Study the drawing (mm; zero at the part's minimum x, y, z) and answer. A direction names the side the tool comes from. Give positions to 0.01 mm unless a question says otherwise; leave off trailing zeros. Write each loop counter-clockwise with the first axis right and the second up, starting at its lowest first coordinate (ties: lowest second). Pieces come first, ordered by that corner, then holes. Notation, with made-up numbers: (19, 30.5) - (46, 30.5) arc R34 cw to (46, 65.5) - close; hole circle Ø7 at (76, -25.75). An arc over 180 degrees is marked (long way). Return JSON: item names as keys, results as strings.
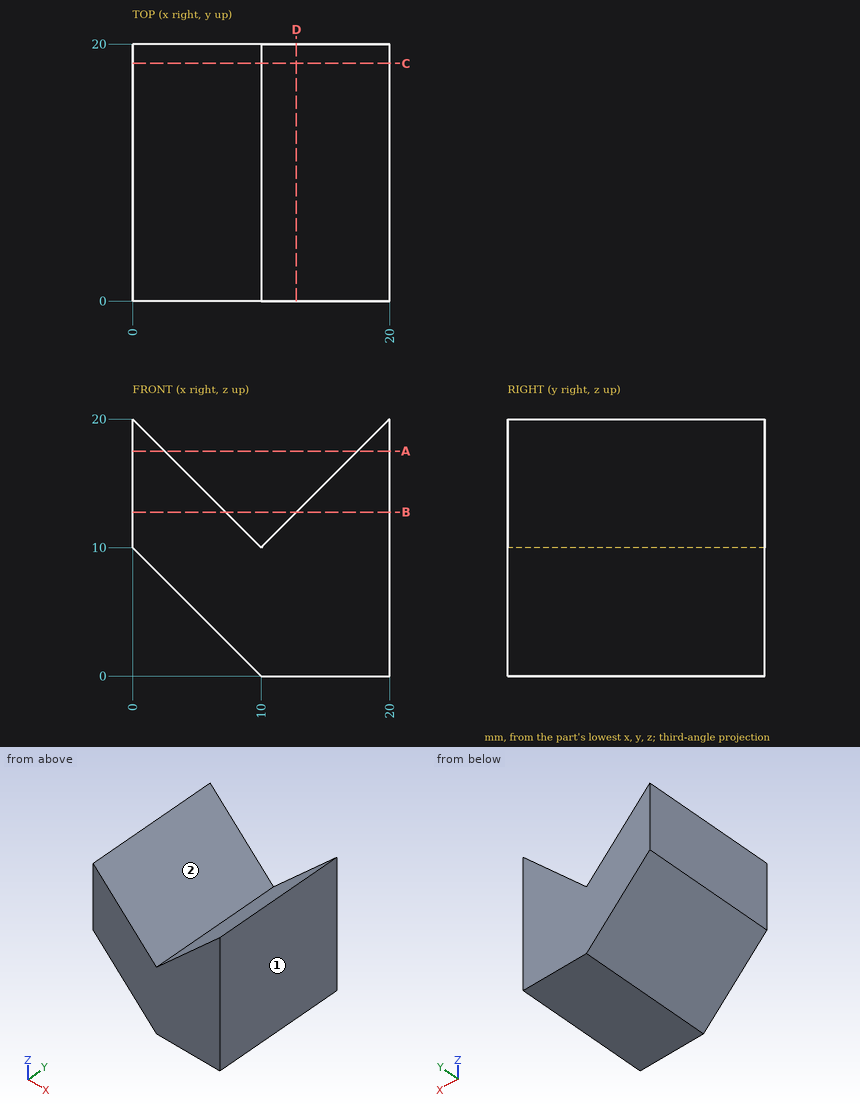
Item 1: A cutting plane is placed at C-C on y = 18.5. Determine the outline of the cut face in (x, z).
Answer below:
{"outline": "(0, 10) - (10, 0) - (20, 0) - (20, 20) - (10, 10) - (0, 20) - close"}
Item 2: A flat-ended cylindrical pin translates along its axis: P1, Ø1.5, axis at x = 6, y = 2.5, coming from the +Z side. Find the tip coordinate at first contact, or state that the pin passes through.
Answer below:
{"P1": "stops at z = 14.75"}
Item 3: A cutting plane is placed at D-D on x = 12.75. Determine the outline of the cut face in (y, z), then the cut area to 3 significant figures.
Answer below:
{"outline": "(0, 0) - (20, 0) - (20, 12.75) - (0, 12.75) - close", "area": "255 mm²"}
Item 4: For the marked faces 1 and 2, determine the directions among +Z, -Z, +X, -X, +Y, -Y from which every point of the face is accessible in a straight line to the end or side of a thin tool.
Answer below:
{"face 1": "+Z, -Z, +X, +Y, -Y", "face 2": "+Z, +Y, -Y"}
Item 5: A cutting plane is placed at A-A on z = 17.5. Determine the outline of the cut face in (x, y), then the cut area to 3 significant figures.
Answer below:
{"outline": "(0, 0) - (2.5, 0) - (2.5, 20) - (0, 20) - close; (17.5, 0) - (20, 0) - (20, 20) - (17.5, 20) - close", "area": "100 mm²"}
Item 6: Consider L1, parallel to X at y = 4.25, z = 17.5; L2, parallel to X at y = 4, z = 12.25; L3, parallel to Z at x = 18, y = 7.75. Determine where each line is inside the solid, lowest interval first.
Answer below:
{"L1": "x = 0 to 2.5, 17.5 to 20", "L2": "x = 0 to 7.75, 12.25 to 20", "L3": "z = 0 to 18"}
Item 7: A cutting plane is placed at B-B on z = 12.75. Determine the outline of the cut face in (x, y), then the cut area to 3 significant figures.
Answer below:
{"outline": "(0, 0) - (7.25, 0) - (7.25, 20) - (0, 20) - close; (12.75, 0) - (20, 0) - (20, 20) - (12.75, 20) - close", "area": "290 mm²"}
